Geometry: see drawing. Coordinates: mm, zero at the bounding-box minimum. A direction names the side the tool comes from. Round coordinates to 2 decimals unless told otherwise and drop trailing zeros. Order: outer loops, then holes, each group sorted by start corner. A loop starts at its lowest first (then second) coordinate and runs counter-clockwise, first axis right, second up. Notation, with made-up numbers: M 36,-12 L 65,-12 A33 ccw 65,24 Z; hole C -10.5,17.25 d11. An arc over 180 degrees is marked long. Answer in a Markdown table with one row per item. Add a question column.
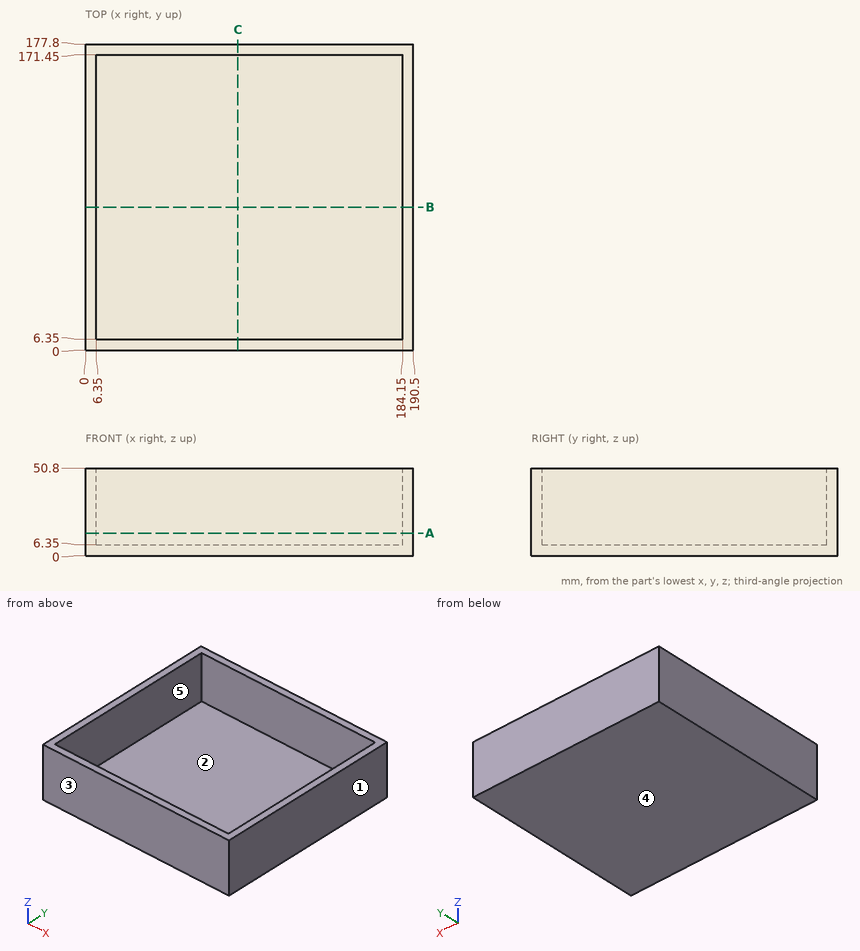
(1) Pin query (flat end, axial travel): pin 1 (12 mm diameter, centred on x = 97.5, y = 158.5, fed in from +Z). Return the tip coordinate at first contact, or that it passes through.
(2) Draft query along Y for the marked faces 3, 4 and 5. Return one class per face: +Y half, -Y half, draft (parallel to the pull), parting line (faces both ways), or undercut.
(3) Cut plane B-B (y = 83). Return loops of the section in (x, z), and give its area (3 significant figures).
(4) Line query: line 1 (X direction, y = 112.5, z = 38); line 2 (Y direction, x = 19, z = 31.5); line 3 (Z direction, x = 145, y = 57). Output: solid intervals per line, ascending. Write a range as from..to.
(5) Access query for the marked faces 1 and 2. Directions: +Z, -Z, +X, -X, +Y, -Y. A direction counts if a zero-diameter tool reaches every point of the face in a straight line with its end or side. Return the directions, or none.
(6) Cut plane A-A (z = 13). Return loops of the section in (x, y), and give its area (3 significant figures).
(7) Cut plane C-C (x = 88.5). Return loops of the section in (y, z), and give its area (3 significant figures).
Answer list:
| question | item | result |
|---|---|---|
| 1 | pin 1 | z = 6.35 |
| 2 | face 3 | -Y half |
| 2 | face 4 | draft |
| 2 | face 5 | undercut |
| 3 | outline | M 0,0 L 190.5,0 L 190.5,50.8 L 184.15,50.8 L 184.15,6.35 L 6.35,6.35 L 6.35,50.8 L 0,50.8 Z |
| 3 | area | 1,770 mm² |
| 4 | line 1 | 0..6.35, 184.15..190.5 |
| 4 | line 2 | 0..6.35, 171.45..177.8 |
| 4 | line 3 | 0..6.35 |
| 5 | face 1 | +Z, -Z, +X, +Y, -Y |
| 5 | face 2 | +Z |
| 6 | outline | M 0,0 L 190.5,0 L 190.5,177.8 L 0,177.8 Z; hole M 6.35,6.35 L 184.15,6.35 L 184.15,171.45 L 6.35,171.45 Z |
| 6 | area | 4,520 mm² |
| 7 | outline | M 0,0 L 177.8,0 L 177.8,50.8 L 171.45,50.8 L 171.45,6.35 L 6.35,6.35 L 6.35,50.8 L 0,50.8 Z |
| 7 | area | 1,690 mm² |
